Verification items for the finished model (mm, model axes). Round coordinates to 2 decimals unless told otherwise and drop trailing zeros. Write each loop counter-clockwise with the first axis right and the second up, starting at its lowest first coordinate (ties: lowest second). Pieces come first, ordered by that corner, then holes. Notation, with made-up numbers: (33, -38) -> (77, -38) arc R19 cw to (77, -16) -> close; hole circle Ø1 at (-14.75, 50.25). An arc over 180 degrees is marked (long way). Answer as a JSON object with one key per item and string values. Group by question number.
(1) Sectioned sample at A-A on z = -210.5. Record the cut outline in (x, y), and give its area (3 significant figures).
(2) Gauge pin test, flat ends, axial feed: pin 1 Ø2 at (y, z) = (-3, -479) entering from -X; pin 2 Ø0.9 at (x, z) = (-7.5, -572.5) entering from -Y; pin 3 Ø6 at (y, z) = (-4.5, -467) entering from -X. Record the tip position at first contact, or that the pin passes through.
(3) Scan lines: L1, parallel to Y at x = 0, z = -462; L2, parallel to X at y = -2, z = -210.5; L3, parallel to X at y = 11.36, z = -252. Record each from-to range of solid material in increasing order. Write a range as from..to.
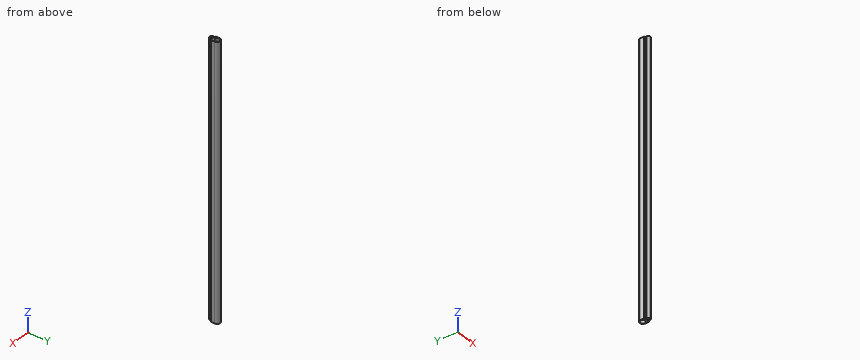
```python
from build123d import *

# Parameters (mm, degrees)
ESQUISSE1_R        = 7
BOSS_EXTRU_1_DEPTH = 796


with BuildPart() as part:
    # Esquisse1 → Boss.-Extru.1 (new body)
    with BuildSketch(Plane.XY.offset(20)):
        with BuildLine():
            Line((-9, 10.864586864), (-9, 0.523924837))
            ThreePointArc((-9, 0.523924837), (-8.854824532, 0.14661401), (-8.478070356, 0))
            Line((-8.478070356, 0), (-5.5, 0))
            ThreePointArc((-5.5, 0), (-4.439339828, -0.439339828), (-4, -1.5))
            Line((-4, -1.5), (-4, -3.5))
            ThreePointArc((-4, -3.5), (-4.292893219, -4.207106781), (-5, -4.5))
            Line((-5, -4.5), (-6.016007613, -4.5))
            ThreePointArc((-6.016007613, -4.5), (-6.227713349, -4.802430523), (-6.174193657, -5.16769643))
            Line((-6.174193657, -5.16769643), (-3.440043573, -9.90338329))
            ThreePointArc((-3.440043573, -9.90338329), (-2.707992766, -10.635434098), (-1.707992766, -10.90338329))
            Line((-1.707992766, -10.90338329), (1.707992766, -10.90338329))
            ThreePointArc((1.707992766, -10.90338329), (2.707992766, -10.635434098), (3.440043573, -9.90338329))
            Line((3.440043573, -9.90338329), (6.174193657, -5.16769643))
            ThreePointArc((6.174193657, -5.16769643), (6.227713349, -4.802430523), (6.016007614, -4.5))
            Line((6.016007614, -4.5), (5, -4.5))
            ThreePointArc((5, -4.5), (4.292893219, -4.207106781), (4, -3.5))
            Line((4, -3.5), (4, -1.5))
            ThreePointArc((4, -1.5), (4.439339828, -0.439339828), (5.5, 0))
            Line((5.5, 0), (8.478070356, 0))
            ThreePointArc((8.478070356, 0), (8.854824532, 0.14661401), (9, 0.523924837))
            Line((9, 0.523924837), (9, 10.864586864))
            ThreePointArc((9, 10.864586864), (0, 19.864586864), (-9, 10.864586864))
        make_face()
        with Locations(Location((0, 11.36, 0), (0, 0, 180))):
            Circle(ESQUISSE1_R, mode=Mode.SUBTRACT)
        with BuildLine():
            Line((1.75, -1.95338329), (1.75, -7.351528839))
            ThreePointArc((1.75, -7.351528839), (0, -9.101528839), (-1.75, -7.351528839))
            Line((-1.75, -7.351528839), (-1.75, -1.95338329))
            ThreePointArc((-1.75, -1.95338329), (0, -0.20338329), (1.75, -1.95338329))
        make_face(mode=Mode.SUBTRACT)
    extrude(amount=-BOSS_EXTRU_1_DEPTH)


solid = part.part
```
Computed values:
{
 "1": {"outline": "(-9, 0.52) arc R0.5 ccw to (-8.48, 0) -> (-5.5, 0) arc R1.5 cw to (-4, -1.5) -> (-4, -3.5) arc R1 cw to (-5, -4.5) -> (-6.02, -4.5) arc R0.5 ccw to (-6.17, -5.17) -> (-3.44, -9.9) arc R2 ccw to (-1.71, -10.9) -> (1.71, -10.9) arc R2 ccw to (3.44, -9.9) -> (6.17, -5.17) arc R0.5 ccw to (6.02, -4.5) -> (5, -4.5) arc R1 cw to (4, -3.5) -> (4, -1.5) arc R1.5 cw to (5.5, 0) -> (8.48, 0) arc R0.5 ccw to (9, 0.52) -> (9, 10.86) arc R9 ccw to (-9, 10.86) -> close; hole circle Ø14 at (0, 11.36); hole (-1.75, -7.35) arc R1.75 ccw to (1.75, -7.35) -> (1.75, -1.95) arc R1.75 ccw to (-1.75, -1.95) -> close", "area": "237 mm2"},
 "2": {"pin 1": "x = -4.13", "pin 2": "y = 0", "pin 3": "x = -6.24"},
 "3": {"L1": "-10.9..-9.1, -0.2..4.36, 18.36..19.86", "L2": "-4..-1.75, 1.75..4", "L3": "-8.99..-7, 7..8.99"}
}
